Can you work these out from the model? Positions are in its coordinate system, mm. Face numbers are marked on the shaded views. Coordinates: 2 decimals unless noted, no trailing zeros. Loops run counter-clockwise (first coordinate to the right, second up) from the corner with the lowest first, then second, coordinate; pieces in that order, holes last.
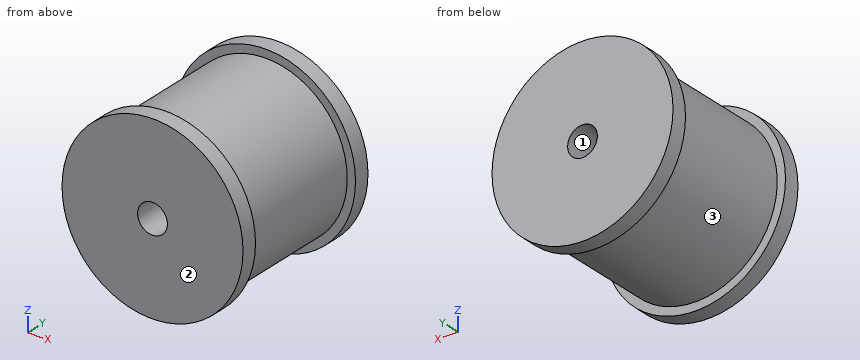
```python
from build123d import *

# Parameters (mm, degrees)
F0_R     = 6.35
F1_DEPTH = 12.7
F2_R     = 6.985
F3_DEPTH = 1.27
F4_R     = 6.985
F5_DEPTH = 1.27
F6_R     = 1.14808
F7_DEPTH = 25.4


with BuildPart() as f1:
    # F0 (on Front) → F1 (new body)
    with BuildSketch(Plane.XZ):
        with Locations((-8.3881383762, 6.6514373757)):
            Circle(F0_R)
    extrude(amount=F1_DEPTH)

    # F2 (on face) → F3 (join)
    with BuildSketch(Plane.XZ.offset(12.7)):
        with Locations((-8.3881383762, 6.6514373757)):
            Circle(F2_R)
    extrude(amount=-F3_DEPTH)

    # F4 (on Front) → F5 (join)
    with BuildSketch(Plane.XZ):
        with Locations((-8.3881383762, 6.6514373757)):
            Circle(F4_R)
    extrude(amount=F5_DEPTH)

    # F6 (on face) → F7 (cut)
    with BuildSketch(Plane.XZ.offset(12.7)):
        with Locations((-8.3881383762, 6.6514373757)):
            Circle(F6_R)
    extrude(amount=-F7_DEPTH, mode=Mode.SUBTRACT)


solid = f1.part
```
Item 1: Suppose I cut it at A-A, the plane z = 7.5. Please give me the cut outline in (x, y).
Results are:
outline: (-15.32, -12.7) - (-9.16, -12.7) - (-9.16, 0) - (-15.32, 0) - (-15.32, -1.27) - (-14.68, -1.27) - (-14.68, -11.43) - (-15.32, -11.43) - close; (-7.61, -12.7) - (-1.45, -12.7) - (-1.45, -11.43) - (-2.1, -11.43) - (-2.1, -1.27) - (-1.45, -1.27) - (-1.45, 0) - (-7.61, 0) - close
Item 2: I need wall thicknesses on line 1 along X through (y, z) = (-11.5, 6.75); line 2 along X through (y, z) = (-2.75, 7); line 3 along Z through (x, y) = (-7.5, -10). Which ranges of each line are inside material? Lowest first, please.
Results are:
line 1: x = -15.37 to -9.53, -7.24 to -1.4
line 2: x = -14.73 to -9.48, -7.29 to -2.05
line 3: z = 0.36 to 5.92, 7.38 to 12.94
Item 3: Suppose I cut it at B-B, the plane x = -3.75. Please give me the cut outline in (y, z).
Results are:
outline: (-12.7, 1.43) - (-11.43, 1.43) - (-11.43, 2.31) - (-1.27, 2.31) - (-1.27, 1.43) - (0, 1.43) - (0, 11.87) - (-1.27, 11.87) - (-1.27, 10.99) - (-11.43, 10.99) - (-11.43, 11.87) - (-12.7, 11.87) - close
Item 4: I'm going to push flat-ended pins straight in: P1, Ø5, axis at x = -12.5, y = -10.5, coming from the -Z side; P2, Ø4, axis at y = -9, z = 11, coming from the -X side; P3, Ø5, axis at y = -6.5, z = 2, coming from the +X side. Where does each tip first touch, or does it pass through?
Results are:
P1: stops at z = -0.1
P2: stops at x = -14.29
P3: stops at x = -2.41
Item 5: We'd pull the mould along Z, two halves only. Please class the marked faces 1, 2 and 3: +Z half, -Z half, draft (parallel to the pull), parting line (faces both ways), or undercut.
Results are:
face 1: undercut
face 2: draft
face 3: parting line
Item 6: Suppose I cut it at D-D, the plane y = -4.75. Please give me the cut outline in (x, z), plus the area to 3 significant figures.
Results are:
outline: circle Ø12.7 at (-8.39, 6.65); hole circle Ø2.3 at (-8.39, 6.65)
area: 123 mm2
Item 7: Suppose I cut it at C-C, the plane z = 4.5. Please give me the cut outline in (x, y).
Results are:
outline: (-15.03, -12.7) - (-1.74, -12.7) - (-1.74, -11.43) - (-2.41, -11.43) - (-2.41, -1.27) - (-1.74, -1.27) - (-1.74, 0) - (-15.03, 0) - (-15.03, -1.27) - (-14.36, -1.27) - (-14.36, -11.43) - (-15.03, -11.43) - close
